```python
from build123d import *

# Parameters (mm, degrees)
SKETCH_1_W           = 160
SKETCH_1_H           = 157.5
EXTRUDE_1_DEPTH      = 46
SKETCH_2_W           = 120
SKETCH_2_H           = 157.5
CUT_EXTRUDE_1_DEPTH  = 43
SKETCH_3_W           = 16
SKETCH_3_H           = 155
CUT_EXTRUDE_2_DEPTH  = 122.31596144
SKETCH_4_R           = 9.5
CUT_EXTRUDE_3_DEPTH  = 171.451056025
SKETCH_5_R           = 9.5
CUT_EXTRUDE_4_DEPTH  = 171.451056025
SKETCH_7_R           = 1.5
CUT_EXTRUDE_6_DEPTH  = 10
SKETCH_10_W          = 16
SKETCH_10_H          = 26
CUT_EXTRUDE_9_DEPTH  = 10
SKETCH_11_W          = 4
SKETCH_11_H          = 26
EXTRUDE_2_DEPTH      = 20
SKETCH_13_R          = 1.5
CUT_EXTRUDE_11_DEPTH = 181.564566014
SKETCH_17_W          = 29.75
SKETCH_17_H          = 3
EXTRUDE_3_DEPTH      = 20
SKETCH_18_R          = 1.5
CUT_EXTRUDE_14_DEPTH = 20
SKETCH_19_W          = 46
SKETCH_19_H          = 27
CUT_EXTRUDE_15_DEPTH = 189.432016919
SKETCH_20_R          = 30
CUT_EXTRUDE_16_DEPTH = 10
SKETCH_21_W          = 120
SKETCH_21_H          = 56.000000256
CUT_EXTRUDE_17_DEPTH = 10
FILLET_1_R           = 60
SKETCH_22_W          = 10
SKETCH_22_H          = 35
CUT_EXTRUDE_18_DEPTH = 10
FILLET_2_R           = 10
SKETCH_24_W          = 31
SKETCH_24_H          = 30
CUT_EXTRUDE_19_DEPTH = 189.432016919
SKETCH_25_W          = 104
SKETCH_25_H          = 21
SKETCH_25_W_2        = 74
SKETCH_25_H_2        = 19.499999744
CUT_EXTRUDE_20_DEPTH = 10


with BuildPart() as part:
    # 草图1 → 凸台-拉伸1 (new body)
    with BuildSketch(Plane.XY):
        Rectangle(SKETCH_1_W, SKETCH_1_H)
    extrude(amount=EXTRUDE_1_DEPTH)

    # 草图2 → 切除-拉伸1 (cut)
    with BuildSketch(Plane.XY.offset(46)):
        Rectangle(SKETCH_2_W, SKETCH_2_H)
    extrude(amount=-CUT_EXTRUDE_1_DEPTH, mode=Mode.SUBTRACT)

    # 草图3 → 切除-拉伸2 (cut, through all)
    with BuildSketch(Plane.XY.offset(46)):
        with Locations((-72, 1.25)):
            Rectangle(SKETCH_3_W, SKETCH_3_H)
        with Locations((72, 1.25)):
            Rectangle(SKETCH_3_W, SKETCH_3_H)
    extrude(amount=-CUT_EXTRUDE_2_DEPTH, mode=Mode.SUBTRACT)

    # 草图4 → 切除-拉伸3 (cut, through all)
    with BuildSketch(Plane.ZY.offset(64)):
        with Locations((31.5, -15.75)):
            Circle(SKETCH_4_R)
    extrude(amount=-CUT_EXTRUDE_3_DEPTH, mode=Mode.SUBTRACT)

    # 草图5 → 切除-拉伸4 (cut, through all)
    with BuildSketch(Plane(origin=(64, 0, 0), x_dir=(0, 0, -1), z_dir=(1, 0, 0))):
        with Locations(Location((-31.5, 29.25, 0), (0, 0, 90))):
            Circle(SKETCH_5_R)
    extrude(amount=-CUT_EXTRUDE_4_DEPTH, mode=Mode.SUBTRACT)

    # 草图7 → 切除-拉伸6 (cut)
    with BuildSketch(Plane.XY.offset(3)):
        with Locations((1, 46.75)):
            Circle(SKETCH_7_R)
        with Locations((18, 46.75)):
            Circle(SKETCH_7_R)
        with Locations((1, 11.75)):
            Circle(SKETCH_7_R)
        with Locations((18, 11.75)):
            Circle(SKETCH_7_R)
    extrude(amount=-CUT_EXTRUDE_6_DEPTH, mode=Mode.SUBTRACT)

    # 草图10 → 切除-拉伸9 (cut)
    with BuildSketch(Plane(origin=(0, -76.25, 0), x_dir=(1, 0, 0), z_dir=(0, 1, 0))):
        with Locations((-72, -13)):
            Rectangle(SKETCH_10_W, SKETCH_10_H)
        with Locations((72, -13)):
            Rectangle(SKETCH_10_W, SKETCH_10_H)
    extrude(amount=-CUT_EXTRUDE_9_DEPTH, mode=Mode.SUBTRACT)

    # 草图11 → 凸台-拉伸2 (add)
    with BuildSketch(Plane.XZ.offset(78.75)):
        with Locations((-62, 13)):
            Rectangle(SKETCH_11_W, SKETCH_11_H)
        with Locations((62, 13)):
            Rectangle(SKETCH_11_W, SKETCH_11_H)
    extrude(amount=EXTRUDE_2_DEPTH)

    # 草图13 → 切除-拉伸11 (cut, through all)
    with BuildSketch(Plane.ZY.offset(64)):
        with Locations(Location((5, -83.75, 0), (0, 0, 270))):
            Circle(SKETCH_13_R)
        with Locations(Location((21, -83.75, 0), (0, 0, 270))):
            Circle(SKETCH_13_R)
        with Locations(Location((21, -93.75, 0), (0, 0, 270))):
            Circle(SKETCH_13_R)
        with Locations(Location((5, -93.75, 0), (0, 0, 270))):
            Circle(SKETCH_13_R)
    extrude(amount=-CUT_EXTRUDE_11_DEPTH, mode=Mode.SUBTRACT)

    # 草图17 → 凸台-拉伸3 (add)
    with BuildSketch(Plane.XY.offset(46)):
        with Locations((-74.875, -77.25)):
            Rectangle(SKETCH_17_W, SKETCH_17_H)
        with Locations((74.875, -77.25)):
            Rectangle(SKETCH_17_W, SKETCH_17_H)
    extrude(amount=-EXTRUDE_3_DEPTH)

    # 草图18 → 切除-拉伸14 (cut)
    with BuildSketch(Plane(origin=(0, -75.75, 0), x_dir=(1, 0, 0), z_dir=(0, 1, 0))):
        with Locations(Location((84.75, -31, 0), (0, 0, 270))):
            Circle(SKETCH_18_R)
        with Locations(Location((84.75, -41, 0), (0, 0, 270))):
            Circle(SKETCH_18_R)
        with Locations(Location((69.75, -31, 0), (0, 0, 270))):
            Circle(SKETCH_18_R)
        with Locations(Location((69.75, -41, 0), (0, 0, 270))):
            Circle(SKETCH_18_R)
        with Locations(Location((-69.75, -31, 0), (0, 0, 270))):
            Circle(SKETCH_18_R)
        with Locations(Location((-69.75, -41, 0), (0, 0, 270))):
            Circle(SKETCH_18_R)
        with Locations(Location((-84.75, -41, 0), (0, 0, 270))):
            Circle(SKETCH_18_R)
        with Locations(Location((-84.75, -31, 0), (0, 0, 270))):
            Circle(SKETCH_18_R)
    extrude(amount=-CUT_EXTRUDE_14_DEPTH, mode=Mode.SUBTRACT)

    # 草图19 → 切除-拉伸15 (cut, through all)
    with BuildSketch(Plane.ZY.offset(64)):
        with Locations((23, 65.25)):
            Rectangle(SKETCH_19_W, SKETCH_19_H)
    extrude(amount=-CUT_EXTRUDE_15_DEPTH, mode=Mode.SUBTRACT)

    # 草图20 → 切除-拉伸16 (cut)
    with BuildSketch(Plane.XY.offset(3)):
        with Locations((5.442e-06, -52.749999744)):
            Circle(SKETCH_20_R)
    extrude(amount=-CUT_EXTRUDE_16_DEPTH, mode=Mode.SUBTRACT)

    # 草图21 → 切除-拉伸17 (cut)
    with BuildSketch(Plane(origin=(0, 0, 0), x_dir=(-1, 0, 0), z_dir=(0, 0, -1))):
        with Locations((0, -50.749999872)):
            Rectangle(SKETCH_21_W, SKETCH_21_H)
    extrude(amount=-CUT_EXTRUDE_17_DEPTH, mode=Mode.SUBTRACT)

    # 圆角1
    fillet_1_edges = [part.edges().sort_by_distance(p)[0] for p in [
        (60, -22.749999744, 1.5),
        (-60, -22.749999744, 1.5),
    ]]
    fillet(fillet_1_edges, radius=FILLET_1_R - 0.0001)  # a hair under: the kernel refuses the full size

    # 草图22 → 切除-拉伸18 (cut)
    with BuildSketch(Plane.XY.offset(3)):
        with Locations((54, -15.75)):
            Rectangle(SKETCH_22_W, SKETCH_22_H)
        with Locations((-54, -15.75)):
            Rectangle(SKETCH_22_W, SKETCH_22_H)
    extrude(amount=-CUT_EXTRUDE_18_DEPTH, mode=Mode.SUBTRACT)

    # 圆角2
    fillet_2_edges = [part.edges().sort_by_distance(p)[0] for p in [
        (62, 51.75, 46),
        (-62, 51.75, 46),
    ]]
    fillet(fillet_2_edges, radius=FILLET_2_R)

    # 草图24 → 切除-拉伸19 (cut, through all)
    with BuildSketch(Plane.ZY.offset(64)):
        with Locations((25.5, -50.75)):
            Rectangle(SKETCH_24_W, SKETCH_24_H)
    extrude(amount=-CUT_EXTRUDE_19_DEPTH, mode=Mode.SUBTRACT)

    # 草图25 → 切除-拉伸20 (cut)
    with BuildSketch(Plane.XY.offset(3)):
        with Locations((0, 29.25)):
            Rectangle(SKETCH_25_W, SKETCH_25_H)
        with Locations((0, -4.999999872)):
            Rectangle(SKETCH_25_W_2, SKETCH_25_H_2)
    extrude(amount=-CUT_EXTRUDE_20_DEPTH, mode=Mode.SUBTRACT)


solid = part.part
```
Could you check a few things on this model? Use its own coordinates, in mm. A direction names the side the tool comes from. Coordinates: 2 decimals unless noted, no trailing zeros. Write each loop counter-clockwise with the first axis right and the second up, starting at its lowest first coordinate (ties: lowest second). Pieces come first, ordered by that corner, then holes. Notation, with made-up numbers: (59, 10.5) -> (101, 10.5) arc R15 ccw to (101, 17.5) -> close; hole circle Ø6 at (-14.75, 5). An arc over 180 degrees is marked (long way). One line per question, with ' | ' between items. Start each with the question number.
1. Please list where these lines run through material, in increasing order: line 1 along X through (y, z) = (-78.1, 41); line 2 along Z through (x, y) = (61.4, -83.75); line 3 along Z through (x, y) = (-69.75, -77.75).
2. If we section it at A-A (x = -23.5): Please give me the cut outline in (y, z).
3. For faces 1 (the face through (-62, -35.75, 25)), 2 (the face through (0, 51.75, 2)), which set-ups out of +Z, -Z, +X, -X, +Y, -Y let a thin tool reach every point of the face, with its end or its side?
4. Will these pins go through, and if not, where does the flat tip stop? P1, Ø11.5, axis at y = -15.75, z = 31.5, coming from the +X side; P2, Ø0.9, axis at x = 78, y = -77, coming from the -Z side; P3, Ø0.9, axis at y = -14.5, z = 1.5, coming from the +X side; P4, Ø16, axis at x = -70, z = 36.5, coming from the -Y side.
5. Thinking about a two-plate mould opening in Z: for faces 3 (the face through (64, -22, 23)), 4 (the face through (62, -35.75, 25)), 5 (the face through (4, 15, 3)), which applies, pulls with the +Z half, pulls with the -Z half, needs draft (parallel to the pull), parting line crosses it, or undercut?
6. If we section it at B-B (y = -56.5): Please give me the cut outline in (x, z).
7. If we section it at C-C (x = 34): Please give me the cut outline in (y, z), and give its area (3 significant figures).
8. If we section it at D-D (x = 76): Please give me the cut outline in (y, z).
Return value:
1) line 1: x = -89.75 to -86.25, -83.25 to -71.25, -68.25 to -60, 60 to 68.25, 71.25 to 83.25, 86.25 to 89.75 | line 2: z = 0 to 3.5, 6.5 to 19.5, 22.5 to 26 | line 3: z = 26 to 29.5, 32.5 to 39.5, 42.5 to 46
2) outline: (-27.54, 0) -> (-14.75, 0) -> (-14.75, 3) -> (-27.54, 3) -> close; (4.75, 0) -> (18.75, 0) -> (18.75, 3) -> (4.75, 3) -> close; (39.75, 0) -> (51.75, 0) -> (51.75, 3) -> (39.75, 3) -> close
3) face 1: +X, -X | face 2: +Z, -Z, +X, -X, +Y
4) P1: passes through | P2: stops at z = 26 | P3: stops at x = 64 | P4: stops at y = -78.75
5) face 3: needs draft | face 4: undercut | face 5: pulls with the +Z half
6) outline: (-64, 0) -> (-53.95, 0) -> (-53.95, 3) -> (-60, 3) -> (-60, 10) -> (-64, 10) -> close; (-64, 41) -> (-60, 41) -> (-60, 46) -> (-64, 46) -> close; (53.95, 0) -> (64, 0) -> (64, 10) -> (60, 10) -> (60, 3) -> (53.95, 3) -> close; (60, 41) -> (64, 41) -> (64, 46) -> (60, 46) -> close
7) outline: (-33.31, 0) -> (-14.75, 0) -> (-14.75, 3) -> (-33.31, 3) -> close; (4.75, 0) -> (18.75, 0) -> (18.75, 3) -> (4.75, 3) -> close; (39.75, 0) -> (51.75, 0) -> (51.75, 3) -> (39.75, 3) -> close | area: 134 mm²
8) outline: (-78.75, 26) -> (-75.75, 26) -> (-75.75, 46) -> (-78.75, 46) -> close
